Model file for the job. Use its own axes, mm. Give positions to 0.01 mm unless a question says otherwise; leave off trailing zeros. Order: outer loops, then holes, each group sorted by start corner. A loop starts at its lowest first (then second) coordinate and runs counter-clockwise, first axis right, second up. Notation, with made-up numbers: M -24,-13.75 L 26,-13.75 A12 cw 26,-3.75 Z; hole C -32.5,72 d9. An arc over 180 degrees is marked long. Return JSON: item names as keys, results as strings. Group by question number.
1. Pin check, flat tips, straight feed: pin 1 (1.5 mm diameter, centred on x = 2, y = 39, fed in from -Z); pin 2 (2.5 mm diameter, centred on y = 40, z = 4.5, fed in from -X). Stop position of each tip, or through.
2. Slice it at B-B on x = 1.9. List the corners of the cut face in (y, z), then the cut area to 3 significant figures.
3. Slice it at A-A on z = 0. List the corners of the cut face in (x, y), then the cut area to 3 significant figures.
4. Slice it at D-D on y = 42.5. List the corners of the cut face in (x, z).
5. Slice it at C-C on z = 4.5. List the corners of the cut face in (x, y), then the cut area to 3 significant figures.
6. Wall check: probe 1 along Z at (x, y) = (1.35, 26.5); probe 2 along Y at (x, z) = (2.2, 3.5); probe 3 along Z at (x, y) = (2.75, 39.5). Give the ranges that are in metal, low to high. Write a range as [from, to].
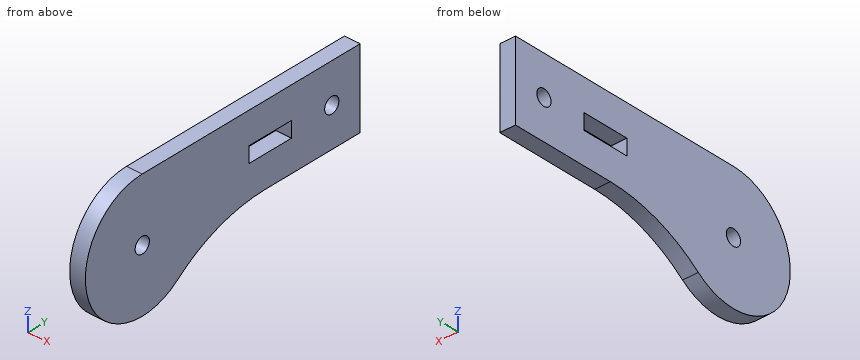
Autodesk Inventor part; units mm, degrees
ref_plane "YZ Plane" through (0, 0, 0) normal (1, 0, 0) x (0, 1, 0)
ref_plane "XZ Plane" through (0, 0, 0) normal (0, 1, 0) x (-1, 0, 0)
ref_plane "XY Plane" through (0, 0, 0) normal (0, 0, 1) x (1, 0, 0)
sketch "Sketch1" plane through (0, 0, 0) normal (1, 0, 0) x (0, 1, 0)
  circle A0 centre (0.0036, 0) radius 1.5
  line L0 (-11.9964, 37.6945) -> (46.0036, 37.6945) construction
  line L1 (0.0036, 12) -> (46.0036, 12)
  line L2 (46.0036, 12) -> (46.0036, -3)
  arc A1 (25.9843, -3) -> (7.4266, -9.4286) centre (25.9843, -33) ccw
  line L3 (25.9843, -3) -> (46.0036, -3)
  arc A2 (25.9843, -3) -> (7.4266, -9.4286) centre (25.9843, -33) ccw
  line L4 (25.9843, -3) -> (46.0036, -3)
  line L5 (46.0036, -3) -> (46.0036, 12)
  line L6 (46.0036, 12) -> (0.0036, 12)
  circle A3 centre (40.0036, 4.5) radius 1.5
  arc A4 (0.0036, 12) -> (7.4266, -9.4286) centre (0.0036, 0) ccw
  circle A5 centre (40.0036, 4.5) radius 1.5
  line L7 (31.5036, 6) -> (22.5036, 6)
  line L8 (22.5036, 6) -> (22.5036, 3)
  line L9 (22.5036, 3) -> (31.5036, 3)
  line L10 (31.5036, 6) -> (31.5036, 3)
  point P0 (0, 0)
  point P1 (1.5, 26.1095)
  point P2 (22.5, 26.1095)
  dimension "d9" = 58
  dimension "d18" = 9
  dimension "d19" = 3
  dimension "d20" = 6
  dimension "d21" = 7.5
  dimension "d22" = 3
  dimension "d23" = 15
  dimension "d24" = 12
  dimension "d25" = 8.5
extrude "Extrusion1" add sketch "Sketch1" along normal blind 3
properties part number "Brazo3Izquierda"
Result:
{
 "1": {"pin 1": "stops at z = -3", "pin 2": "passes through"},
 "2": {"outline": "M 0,12 A12 ccw long 7.43,-9.43 A30 cw 25.98,-3 L 46,-3 L 46,12 Z; hole C 0,0 d3; hole M 22.5,3 L 31.5,3 L 31.5,6 L 22.5,6 Z; hole C 40,4.5 d3", "area": "974 mm2"},
 "3": {"outline": "M 0,-12 L 3,-12 L 3,-1.5 L 0,-1.5 Z; M 0,1.5 L 3,1.5 L 3,46 L 0,46 Z", "area": "165 mm2"},
 "4": {"outline": "M 0,-3 L 3,-3 L 3,12 L 0,12 Z"},
 "5": {"outline": "M 0,-11.12 L 3,-11.12 L 3,22.5 L 0,22.5 Z; M 0,31.5 L 3,31.5 L 3,38.5 L 0,38.5 Z; M 0,41.5 L 3,41.5 L 3,46 L 0,46 Z", "area": "135 mm2"},
 "6": {"probe 1": "z = [-3, 3], [6, 12]", "probe 2": "y = [-11.47, 22.5], [31.5, 38.89], [41.12, 46]", "probe 3": "z = [-3, 3.09], [5.91, 12]"}
}
